```python
from build123d import *

# Parameters (mm, degrees)
F1_DEPTH = 15
F2_R     = 2
F3_R     = 1.5
F4_DEPTH = 30.001


with BuildPart() as f1:
    # F0 (on Front) → F1 (new body, symmetric)
    with BuildSketch(Plane.XZ):
        with BuildLine():
            ThreePointArc((-14.510562, 21), (-17.890873, 17.890873), (-21, 14.510562))
            Line((-21, 14.510562), (-21, -14.510562))
            ThreePointArc((-21, -14.510562), (-17.890873, -17.890873), (-14.510562, -21))
            Line((-14.510562, -21), (14.510562, -21))
            ThreePointArc((14.510562, -21), (17.890873, -17.890873), (21, -14.510562))
            Line((21, -14.510562), (21, 14.510562))
            ThreePointArc((21, 14.510562), (17.890873, 17.890873), (14.510562, 21))
            Line((14.510562, 21), (-14.510562, 21))
        make_face()
    extrude(amount=F1_DEPTH, both=True)

    # F2
    f2_edges = [f1.edges().sort_by_distance(p)[0] for p in [
        (14.510562, 0, 21),
        (21, 0, 14.510562),
        (21, 0, -14.510562),
        (14.510562, 0, -21),
        (-14.510562, 0, -21),
        (-21, 0, -14.510562),
        (-21, 0, 14.510562),
        (-14.510562, 0, 21),
    ]]
    fillet(f2_edges, radius=F2_R)

    # F3 (on face) → F4 (cut, through all)
    with BuildSketch(Plane.XZ.offset(15)):
        with Locations((15.5, 15.5)):
            Circle(F3_R)
        with Locations((-15.5, 15.5)):
            Circle(F3_R)
        with Locations((-15.5, -15.5)):
            Circle(F3_R)
        with Locations((15.5, -15.5)):
            Circle(F3_R)
    extrude(amount=-F4_DEPTH, mode=Mode.SUBTRACT)


solid = f1.part
```
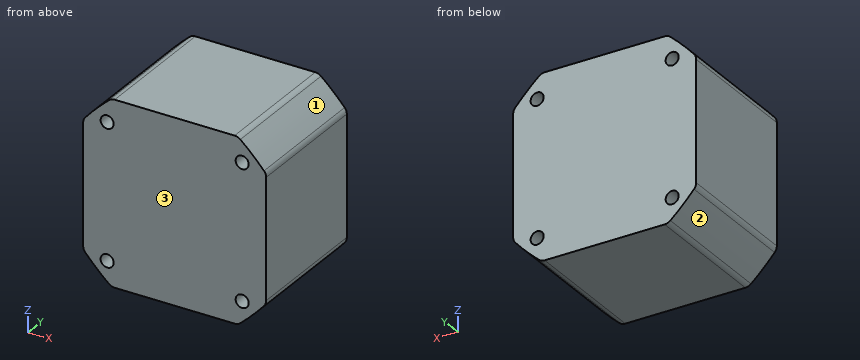
The listing builds one solid part. Answer for the finished solid, in the listing's coordinates (mm). Face numbers are marked on the shaded views. Round coordinates to 2 decimals unless told otherwise and drop trailing zeros. Write each loop counter-clockwise with the first axis right and the second up, starting at its lowest first coordinate (ties: lowest second). Pieces come first, ordered by that corner, then holes. Notation, with made-up numbers: (23.5, 60.5) -> (82.5, 60.5) arc R26 cw to (82.5, 92.5) -> close; hole circle Ø3 at (7.25, 70). An arc over 180 degrees is marked (long way). Answer as a JSON object with one key per item and string values. Group by question number.
Q1. Each of these flat-tipped pins is pushed along its axis until it touches: pin 1 Ø4 at (x, z) = (-15.5, -15.5) entering from -Y; pin 2 Ø3 at (x, y) = (15.5, -4) entering from +Z; pin 3 Ø2 at (y, z) = (9.5, -15) entering from +X. Where does it stop, or does it pass through?
Q2. Section B-B (x = 18) is taken. Write down the section's boundary in (y, z), plus the area to 3 significant figures.
Q3. Section A-A (y = 2.75) is taken. Write down the section's boundary in (x, z), plus the area to 3 significant figures.
Q4. Straight lines are drawn through the part: line 1 along Z through (x, y) = (15.5, -4.25); line 2 along Z through (x, y) = (-16, -8). For each, find the intervals that lie inside material, in ascending order.
Q5. Determine the mould class of the marked faces 1, 2 and 3 for opening direction X: pulls with the +X half, pulls with the -X half, needs draft (parallel to the pull), parting line crosses it, or undercut.
Check values:
{
 "1": {"pin 1": "y = -15", "pin 2": "z = 20.99", "pin 3": "x = 20.99"},
 "2": {"outline": "(-15, -17.78) -> (15, -17.78) -> (15, 17.78) -> (-15, 17.78) -> close", "area": "1,070 mm^2"},
 "3": {"outline": "(-21, -13.77) arc R2 ccw to (-20.51, -15.08) arc R55 ccw to (-15.08, -20.51) arc R2 ccw to (-13.77, -21) -> (13.77, -21) arc R2 ccw to (15.08, -20.51) arc R55 ccw to (20.51, -15.08) arc R2 ccw to (21, -13.77) -> (21, 13.77) arc R2 ccw to (20.51, 15.08) arc R55 ccw to (15.08, 20.51) arc R2 ccw to (13.77, 21) -> (-13.77, 21) arc R2 ccw to (-15.08, 20.51) arc R55 ccw to (-20.51, 15.08) arc R2 ccw to (-21, 13.77) -> close; hole circle Ø3 at (-15.5, -15.5); hole circle Ø3 at (-15.5, 15.5); hole circle Ø3 at (15.5, -15.5); hole circle Ø3 at (15.5, 15.5)", "area": "1,660 mm^2"},
 "4": {"line 1": "-20.14 to -17, -14 to 14, 17 to 20.14", "line 2": "-19.69 to -16.91, -14.09 to 14.09, 16.91 to 19.69"},
 "5": {"face 1": "pulls with the +X half", "face 2": "pulls with the -X half", "face 3": "needs draft"}
}
